```python
from build123d import *

# Parameters (mm, degrees)
EXTRU_MINCE1_DEPTH      = 32
BOSS_EXTRU_1_DEPTH      = 1
ESQUISSE3_R             = 1.2
BOSS_EXTRU_2_DEPTH      = 32
CONG_1_R                = 2
ENL_V_MAT_EXTRU_1_DEPTH = 83.37492882


with BuildPart() as part:
    # Esquisse1 → Extru.-Mince1 (new body)
    with BuildSketch(Plane(origin=(0, 0, 0), x_dir=(1, 0, 0), z_dir=(0, 1, 0))):
        with BuildLine():
            Line((-76, 30), (-76, 14))
            ThreePointArc((-76, 14), (-71.899494937, 4.100505063), (-62, 0))
            Line((-62, 0), (0, 0))
            ThreePointArc((0, 0), (12.124355653, 7), (12.124355653, 21))
            Line((12.124355653, 21), (6.92820323, 30))
            Line((6.92820323, 30), (7.794228634, 30.5))
            Line((7.794228634, 30.5), (12.990381057, 21.5))
            ThreePointArc((12.990381057, 21.5), (12.990381057, 6.5), (0, -1))
            Line((0, -1), (-62, -1))
            ThreePointArc((-62, -1), (-72.606601718, 3.393398282), (-77, 14))
            Line((-77, 14), (-77, 30))
            Line((-77, 30), (-76, 30))
        make_face()
    extrude(amount=EXTRU_MINCE1_DEPTH)

    # Esquisse2 → Boss.-Extru.1 (add)
    with BuildSketch(Plane(origin=(0, 0, 0), x_dir=(1, 0, 0), z_dir=(0, 1, 0))):
        with BuildLine():
            Line((-76, 30), (6.92820323, 30))
            Line((6.92820323, 30), (12.124355653, 21))
            ThreePointArc((12.124355653, 21), (12.124355653, 7), (0, 0))
            Line((0, 0), (-62, 0))
            ThreePointArc((-62, 0), (-71.899494937, 4.100505063), (-76, 14))
            Line((-76, 14), (-76, 30))
        make_face()
    extrude(amount=BOSS_EXTRU_1_DEPTH)

    # Esquisse3 → Boss.-Extru.2 (add)
    # profile 1 of 2: a face of its own
    with BuildSketch(Plane(origin=(0, 0, 0), x_dir=(1, 0, 0), z_dir=(0, 1, 0))):
        with BuildLine():
            Line((-11.236067977, -1), (-6.763932023, -1))
            ThreePointArc((-6.763932023, -1), (-9, -6), (-11.236067977, -1))
        make_face()
        with Locations(Location((-9, -3, 0), (0, 0, 270))):
            Circle(ESQUISSE3_R, mode=Mode.SUBTRACT)
    # profile 2 of 2: a face of its own
    with BuildSketch(Plane(origin=(0, 0, 0), x_dir=(1, 0, 0), z_dir=(0, 1, 0))):
        with BuildLine():
            ThreePointArc((-70.465946464, 1.617441683), (-70.268656396, -3.71854942), (-66.052301711, -0.442259201))
            ThreePointArc((-66.052301711, -0.442259201), (-68.34328198, 0.4072529), (-70.465946464, 1.617441683))
        make_face()
        with Locations(Location((-69, -1, 0), (0, 0, 270))):
            Circle(ESQUISSE3_R, mode=Mode.SUBTRACT)
    extrude(amount=BOSS_EXTRU_2_DEPTH)

    # Congé1
    cong_1_edges = [part.edges().sort_by_distance(p)[0] for p in [
        (-6.763932023, 16, 1),
        (-11.236067977, 16, 1),
        (-70.465946464, 16, -1.617441683),
        (-66.052301711, 16, 0.442259201),
    ]]
    fillet(cong_1_edges, radius=CONG_1_R)

    # Esquisse4 → Enlèv. mat.-Extru.1 (cut, through all)
    with BuildSketch(Plane(origin=(-7.939310229, 0, 1), x_dir=(-1, 0, 0), z_dir=(0, 0, -1))):
        with BuildLine():
            Line((-22.939310229, 32), (-7.939310229, 32))
            Line((-7.939310229, 32), (-7.939310229, 30))
            ThreePointArc((-7.939310229, 30), (-9.403776323, 26.464466094), (-12.939310229, 25))
            Line((-12.939310229, 25), (-22.939310229, 25))
            Line((-22.939310229, 25), (-22.939310229, 32))
        make_face()
    extrude(amount=ENL_V_MAT_EXTRU_1_DEPTH, mode=Mode.SUBTRACT)


solid = part.part
```
Verification items for the finished model (mm, model axes). A direction names the side the tool comes from. Give positions to 0.01 mm unless a question says otherwise; leave off trailing zeros. Loops run counter-clockwise (first coordinate to the right, second up) from the corner with the lowest first, then second, coordinate; pieces in that order, holes last.
1. Set-up check for faces 1 (the cylindrical face through (-12.6, 16.22, 1.57)), 2 (the flat face through (-31, 16, 0)), 3 (the cylindrical face through (12.02, 12.07, -6.82)): record each of +Z, -Z, +X, -X, +Y, -Y from which the full face is reachable in a straight line by a thin tool's end or side.
2. Section check B-B, the plane x = -21. Enter the section's corners in (y, z), then the cut area to 3 significant figures.
3. Section check D-D, the plane x = -9. Enter the section's corners in (y, z), then the cut area to 3 significant figures.
4. Mould release check, pull along Z, two halves, no side actions. Record for faces 4 (the cylindrical face through (-10.17, 15.78, 2.74)), 5 (the flat face through (-38, 16, 1)), 6 (the flat face through (-67, 32, 0)), 7 (the flat face through (-35.2, 0.5, -30)): released by +Z, released by -Z, zero draft, split by the parting line, or undercut.
5. Go/stop test with flat-tipped pins: pin 1 Ø4 at (y, z) = (21.5, -21.5) entering from +X; pin 2 Ø9 at (x, z) = (-17.5, -14) entering from +Y; pin 3 Ø16 at (x, y) = (-23.5, 21) entering from -Z. Record where each tip stops, or that it passes through.
6. Thickness scan on line 1 (Z direction, x = -21, y = 14); line 2 (X direction, y = 12.5, z = -28). Record the ranges inside material, lowest first.
7. Section check A-A, the plane x = -69. Enter the section's corners in (y, z), then the cut area to 3 significant figures.
8. Section check C-C, the plane z = -15.5. Enter the section's corners in (x, y), then the cut area to 3 significant figures.
Geometry says:
1. face 1: +Z, +Y, -Y
1. face 2: -Z, +Y
1. face 3: +Y
2. outline: (0, -30) - (1, -30) - (1, 0) - (32, 0) - (32, 1) - (0, 1) - close
2. area: 62.0 mm2
3. outline: (0, -30) - (1, -30) - (1, 0) - (32, 0) - (32, 1.8) - (0, 1.8) - close; (0, 4.2) - (32, 4.2) - (32, 6) - (0, 6) - close
3. area: 145 mm2
4. face 4: undercut
4. face 5: released by +Z
4. face 6: zero draft
4. face 7: released by -Z
5. pin 1: stops at x = 13.96
5. pin 2: stops at y = 1
5. pin 3: stops at z = 0
6. line 1: z = 0 to 1
6. line 2: x = -77 to -76, 8.08 to 9.24
7. outline: (0, -30) - (1, -30) - (1, -1.88) - (32, -1.88) - (32, -0.2) - (0, -0.2) - close; (0, 2.2) - (32, 2.2) - (32, 4) - (0, 4) - close
7. area: 139 mm2
8. outline: (-77, 0) - (14.92, 0) - (14.92, 25) - (13.92, 25) - (13.92, 1) - (-76, 1) - (-76, 32) - (-77, 32) - close
8. area: 147 mm2
